Input: dimensioned drawing with shaded views. Units: mm. Origin: part minimum x, y, z. Round coordinates to 2 decimals unless told otherwise and drop trailing zeros. Write each loop counter-clockwise with the first axis right and the second up, starting at its lowest first coordinate (ties: lowest second). Pieces come first, ordered by that corner, then holes. Notation, with made-up numbers: (78.25, 9.5) - (86.25, 9.5) arc R22 cw to (86.25, 43.5) - close; hole circle Ø5 at (62, 5.25). An arc over 180 degrees is marked (long way). Use one line per item in the form item = value.
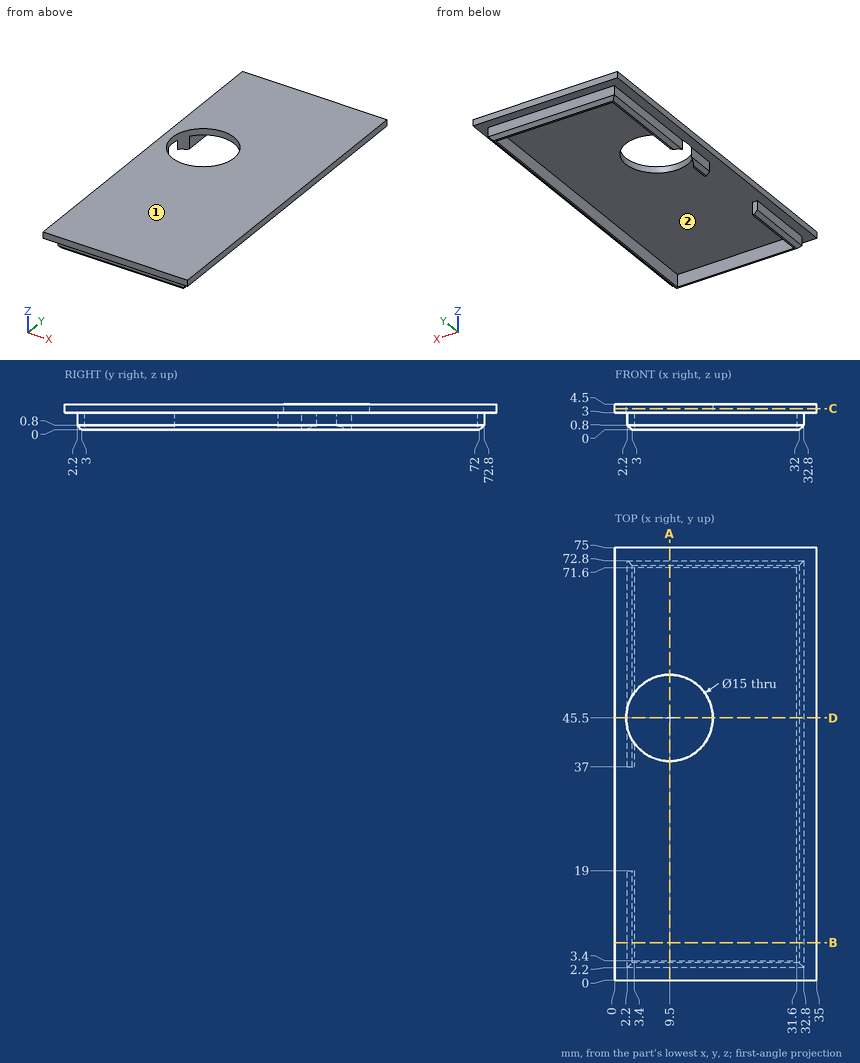
(1) Cut plane D-D on y = 45.5. Output: boundary loops of the cut face in (x, z), then the cut area to 3 significant figures.
Derived:
outline = (0, 3) - (2, 3) - (2, 4.5) - (0, 4.5) - close; (17, 3) - (31.6, 3) - (31.6, 0) - (32, 0) - (32.8, 0.8) - (32.8, 3) - (35, 3) - (35, 4.5) - (17, 4.5) - close
area = 33.3 mm^2
(2) Draft query along X for the marked faces 1 and 2. Return one class per face: released by +X, released by -X, zero draft, split by the parting line, or undercut.
Derived:
face_1 = zero draft
face_2 = undercut
(3) Cut plane C-C on z = 3.7. Output: boundary loops of the cut face in (x, y).
Derived:
outline = (0, 0) - (35, 0) - (35, 75) - (0, 75) - close; hole circle Ø15 at (9.5, 45.5)
(4) Material intervals for L1, parallel to X at y = 16, z = 1.5; L2, parallel to Y at x = 9.5, z = 2.4; L3, parallel to X at y = 45.5, z = 3.35, sorted ascending.
Derived:
L1 = 2.2 to 3.4, 31.6 to 32.8
L2 = 2.2 to 3.4, 71.6 to 72.8
L3 = 0 to 2, 17 to 35
(5) First-contact query: pin 1 Ø1 at (x, z) = (3, 1.5) entering from +Y; pin 2 Ø0.7 at (y, z) = (43, 2.5) entering from +X; pin 3 Ø1.5 at (x, z) = (18, 2) entering from -Y. Flat tips, straight axial feed; report the tip coordinate or a pass-through.
Derived:
pin_1 = 72.8
pin_2 = 32.8
pin_3 = 2.2
(6) Cut plane B-B on y = 6.5. Output: boundary loops of the cut face in (x, z), then the cut area to 3 significant figures.
Derived:
outline = (0, 3) - (2.2, 3) - (2.2, 0.8) - (3, 0) - (3.4, 0) - (3.4, 3) - (31.6, 3) - (31.6, 0) - (32, 0) - (32.8, 0.8) - (32.8, 3) - (35, 3) - (35, 4.5) - (0, 4.5) - close
area = 59.1 mm^2
(7) Cut plane A-A on x = 9.5. Output: boundary loops of the cut face in (y, z).
Derived:
outline = (0, 3) - (2.2, 3) - (2.2, 0.8) - (3, 0) - (3.4, 0) - (3.4, 3) - (38, 3) - (38, 4.5) - (0, 4.5) - close; (53, 3) - (71.6, 3) - (71.6, 0) - (72, 0) - (72.8, 0.8) - (72.8, 3) - (75, 3) - (75, 4.5) - (53, 4.5) - close
